Model file for the job. Use its own axes, mm. Face numbers are marked on the shaded views. A direction names the side the tool comes from. Coordinates: 2 decimals unless noted, no trailing zeros. Order: outer loops, then holes, each group sorted by start corner. A loop starts at its lowest first (then second) coordinate and runs counter-clockwise, first axis right, second up. Notation, with made-up numbers: (-25, 60) -> (-9, 60) arc R28 cw to (-9, 95) -> close; hole circle Ø3 at (24, 17). An arc over 180 degrees is marked (long way). Use CSV: the item, a comma, the result in double quotes. Start each with the question number.
(1) Tool access for the marked faces 4 and 5: list every direction of +Z, -Z, +X, -X, +Y, -Y with a clear straight run to the whole face (end or side of a thin tool).
(2) Cut at D-D on x = 1. Write the cut outline in (y, z) (3 decimals).
(3) Cut at C-C on z = 0. Write the cut outline in (x, y) (3 decimals), plus the area to 3 significant figures.
(4) Probe L1, parallel to Z at x = 0, y = 0.2; L2, parallel to X at y = 0.2, z = 0; L3, parallel to Y at x = 0.75, z = -1.1. List the from-to ranges inside material, lowest first.
(5) Pull direction Z, two halves, no side cores. Call the marked faces 1, 2 and 3: pulls with the +Z half, pulls with the -Z half, needs draft (parallel to the pull), parting line crosses it, or undercut.
(6) Cut at A-A on x = 0. Write the cut outline in (y, z) (3 decimals), plus the area to 3 significant figures.
```python
from build123d import *

# Parameters (mm, degrees)
BOSS_EXTRUDE1_DEPTH   = 2
BOSS_EXTRUDE1_2_DEPTH = 2
BOSS_EXTRUDE2_DEPTH   = 0.5
HOLE2_OUTLINE_R       = 0.5
HOLE2_DEPTH           = 0.5
FILLET2_R             = 0.125
FILLET3_R             = 0.125


# Read off the part's stored shape, not the designer's step: Hole2
with BuildPart() as part:
    # Sketch1 → Boss-Extrude1 (new body)
    with BuildSketch(Plane(origin=(0, 0, 0), x_dir=(1, 0, 0), z_dir=(0, 1, 0))):
        with BuildLine():
            Line((-1.0392304845412224, 2.6), (-1.5, 2.6))
            ThreePointArc((-1.5, 2.6), (-4.1, -1.7e-16), (-1.4999999999999993, -2.6))
            Line((-1.5, -2.6), (-1.039230484541227, -2.6))
            ThreePointArc((-1.0392304845412341, -2.6000000000000365), (-2.8, 2.83e-15), (-1.0392304845412292, 2.6000000000000387))
        make_face()
    extrude(amount=BOSS_EXTRUDE1_DEPTH)



with BuildPart() as body_2:
    # Sketch1 → Boss-Extrude1 2 (new body)
    with BuildSketch(Plane(origin=(0, 0, 0), x_dir=(1, 0, 0), z_dir=(0, 1, 0))):
        with BuildLine():
            Line((1.4999999999999991, 2.6000000000000005), (1.039230484541188, 2.6000000000000005))
            ThreePointArc((1.0392304845411973, 2.6000000000000516), (2.8000000000000003, 3.11e-15), (1.039230484541203, -2.6000000000000494))
            Line((1.0392304845411937, -2.5999999999999996), (1.5000000000000009, -2.5999999999999996))
            ThreePointArc((1.5000000000000009, -2.5999999999999996), (4.1, 1.73e-15), (1.4999999999999984, 2.6000000000000005))
        make_face()
    extrude(amount=BOSS_EXTRUDE1_2_DEPTH)


with BuildPart() as part_1:
    add(part.part)

    add(body_2.part)  # Boss-Extrude2 merges body 2
    # Sketch1<3> → Boss-Extrude2 (add)
    with BuildSketch(Plane(origin=(0, 0, 0), x_dir=(1, 0, 0), z_dir=(0, 1, 0))):
        with BuildLine():
            Line((1.0392304845411884, 2.6000000000000005), (-1.0392304845412224, 2.6))
            ThreePointArc((-1.0392304845412292, 2.6000000000000387), (-2.8, 2.83e-15), (-1.0392304845412341, -2.6000000000000365))
            Line((-1.039230484541227, -2.6), (1.0392304845411937, -2.5999999999999996))
            ThreePointArc((1.039230484541203, -2.600000000000049), (2.3183879481997147, -1.5700564708450193), (2.8, -6.9e-16))
            ThreePointArc((2.8, 0), (2.318387948199713, 1.5700564708450213), (1.0392304845411973, 2.6000000000000516))
        make_face()
    extrude(amount=BOSS_EXTRUDE2_DEPTH)

    # Hole2 outline → Hole2 (cut)
    with BuildSketch(Plane(origin=(0, 0, 0), x_dir=(1, 0, 0), z_dir=(0, 1, 0))):
        Circle(HOLE2_OUTLINE_R)
    extrude(amount=HOLE2_DEPTH, mode=Mode.SUBTRACT)

    # Fillet2
    # the kernel refuses this fillet: 0.125 mm, written as the material it takes off along each edge
    with BuildSketch(Plane(origin=(1.4999999999999987, 0, -2.6000000000000005), x_dir=(0, 1, 3.55e-15), z_dir=(-1, 0, 1.5e-16))) as fillet2_piece_1:
        with BuildLine():
            CenterArc((FILLET2_R, -FILLET2_R), FILLET2_R, 90.00000000000021, 89.99999999999979)
            Line((4.3e-16, -FILLET2_R), (0, 0))
            Line((0, 0), (FILLET2_R, 0))
        make_face()
    extrude(amount=2.9999999999999987, mode=Mode.SUBTRACT)
    with BuildSketch(Plane(origin=(1.4999999999999996, 0, -3.3e-16), x_dir=(5.1e-16, 0, 1), z_dir=(-1, 0, 5.1e-16))) as fillet2_piece_2:
        with BuildLine():
            CenterArc((2.6 - FILLET2_R, FILLET2_R), FILLET2_R, 270, 90)
            Line((2.6, FILLET2_R), (2.6, 0))
            Line((2.6, 0), (2.6 - FILLET2_R, 0))
        make_face()
    revolve(axis=Axis((1.4999999999999996, 0, -3.3e-16), (0, 1, 0)), revolution_arc=180, mode=Mode.SUBTRACT)
    with BuildSketch(Plane(origin=(1.5000000000000009, 0, 2.5999999999999996), x_dir=(-1.5e-16, 0, -1), z_dir=(-1, 0, 1.5e-16))) as fillet2_piece_3:
        with BuildLine():
            CenterArc((FILLET2_R, -FILLET2_R), FILLET2_R, 90, 90)
            Line((0, -FILLET2_R), (0, 0))
            Line((0, 0), (FILLET2_R, 0))
        make_face()
    extrude(amount=3.0000000000000004, mode=Mode.SUBTRACT)
    with BuildSketch(Plane(origin=(-1.0392304845412306, 0.5, 2.6000000000000183), x_dir=(-0.8909362232588717, 0, -0.4541284466813525), z_dir=(0, 1, 0))) as fillet2_piece_4:
        with BuildLine():
            CenterArc((0.5210688048998693, 0.1244811743822189), FILLET2_R, 115.6197462863135, 149.1581720450634)
            Line((0.4670192388207316, 0.23719161935808136), (0.46161428221281786, 0.24846266385566762))
            ThreePointArc((0.46161428221281786, 0.24846266385566762), (0.404839646312147, 0.2203852471241299), (-0.00567660558351699, 0.01113670279073605))
            Line((-0.00567660558351699, 0.01113670279073605), (0.00113770481419139, -0.01244811743822212))
            ThreePointArc((0.00113770481419139, -0.01244811743822212), (0.254845878378973, -0.00087830616170155), (0.5085540519437544, -0.0124481174382219))
            Line((0.5085540519437544, -0.0124481174382219), (0.5096917567579465, -1e-17))
        make_face()
    extrude(amount=2.809500939581575, mode=Mode.SUBTRACT)
    with BuildSketch(Plane(origin=(1.0392304845411986, 0.5, 2.600000000000024), x_dir=(0.8909362232588801, 0, -0.45412844668133606), z_dir=(0, 1, 0))) as fillet2_piece_5:
        with BuildLine():
            CenterArc((0.5210688048999061, -0.12448117438221841), FILLET2_R, 95.22208166862436, 149.158172045063)
            Line((0.4670192388207701, -0.23719161935808164), (0.46161428221285655, -0.248462663855668))
            ThreePointArc((0.46161428221285655, -0.248462663855668), (0.4048396463121838, -0.22038524712413216), (-0.00567660558351678, -0.01113670279073616))
            Line((-0.00567660558351678, -0.01113670279073616), (0.00113770481419136, 0.01244811743822204))
            ThreePointArc((0.00113770481419136, 0.01244811743822204), (0.2548458783789898, 0.00087830616169669), (0.5085540519437883, 0.0124481174382219))
            Line((0.5085540519437883, 0.0124481174382219), (0.5096917567579807, 2e-17))
        make_face()
    extrude(amount=2.8095009395816612, mode=Mode.SUBTRACT)
    with BuildSketch(Plane(origin=(1.0392304845411924, 0.5, -2.600000000000026), x_dir=(0.9999989359619427, 0, 0.001458792302720678), z_dir=(0, 1, 0))) as fillet2_piece_6:
        with BuildLine():
            CenterArc((0.5209523714738641, -0.12496755127300935), FILLET2_R, 88.69445799122111, 149.1581720450468)
            Line((0.45444002573679215, -0.23080283775418345), (0.447788791163085, -0.24138636640230085))
            ThreePointArc((0.447788791163085, -0.24138636640230085), (0.22682229100640774, -0.11618451467849848), (-0.00462248445880959, -0.01161389845952106))
            Line((-0.00462248445880959, -0.01161389845952106), (-1.823490378401e-05, 0.01249998669952446))
            ThreePointArc((-1.823490378401e-05, 0.01249998669952446), (0.46075079027872196, 0.01317215372197879), (0.5240851762685466, 0.01249675512730089))
            Line((0.5240851762685466, 0.01249675512730089), (0.5238003758326663, 0))
        make_face()
    extrude(amount=2.8095009395816657, mode=Mode.SUBTRACT)
    with BuildSketch(Plane(origin=(-1.4999999999999996, 0, 0), x_dir=(-1.7e-16, 0, -1), z_dir=(1, 0, -1.7e-16))) as fillet2_piece_7:
        with BuildLine():
            CenterArc((2.6 - FILLET2_R, FILLET2_R), FILLET2_R, 270, 90)
            Line((2.6 - FILLET2_R, -1e-17), (2.6, 0))
            Line((2.6, 0), (2.6, FILLET2_R))
        make_face()
    revolve(axis=Axis((-1.4999999999999996, 0, 0), (0, 1, 0)), revolution_arc=180, mode=Mode.SUBTRACT)
    with BuildSketch(Plane(origin=(-1.0392304845412257, 0.5, -2.600000000000019), x_dir=(-0.9999989359619427, 0, 0.0014587923027088937), z_dir=(0, 1, 0))) as fillet2_piece_8:
        with BuildLine():
            CenterArc((0.5209523714738317, 0.1249675512730093), FILLET2_R, 122.14736996373313, 149.15817204504657)
            Line((0.4544400257367579, 0.23080283775418217), (0.44778879116305065, 0.24138636640229952))
            ThreePointArc((0.44778879116305065, 0.24138636640229952), (0.2268222910063884, 0.11618451467850208), (-0.00462248445880995, 0.01161389845952101))
            Line((-0.00462248445880995, 0.01161389845952101), (-1.823490378386e-05, -0.01249998669952446))
            ThreePointArc((-1.823490378386e-05, -0.01249998669952446), (0.46075079027869037, -0.01317215372197953), (0.524085176268516, -0.01249675512730089))
            Line((0.524085176268516, -0.01249675512730089), (0.5238003758326356, 0))
        make_face()
    extrude(amount=2.809500939581589, mode=Mode.SUBTRACT)

    # Fillet3
    fillet3_edges = [part_1.edges().sort_by_distance(p)[0] for p in [
        (4.1, 2, 5.853e-14),
        (-2.799999999999999, 2, -1.78e-15),
        (-4.1, 2, 6.033e-14),
        (-1.440341394717322, 2, -2.510422560661599),
        (-1.4403413947172043, 2, 2.5104225606616026),
        (2.8, 2, -2.2e-16),
        (1.4403413947173214, 2, -2.5104225606615973),
        (1.4403413947172052, 2, 2.510422560661605),
    ]]
    fillet(fillet3_edges, radius=FILLET3_R)


solid = part_1.part
```
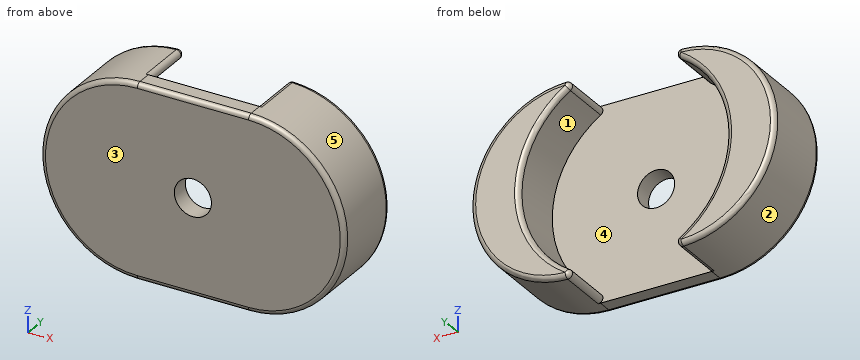
Outcome:
1,face 4,"+Y"
1,face 5,"+X, +Y, -Y"
2,outline,"(0, -2.475) arc R0.125 ccw to (0.125, -2.6) -> (0.5, -2.6) -> (0.5, 2.6) -> (0.125, 2.6) arc R0.125 ccw to (0, 2.475) -> close"
3,outline,"(-4.1, 0.125) arc R0.125 ccw to (-3.975, 0) -> (-0.5, 0) -> (-0.5, 0.5) -> (-2.8, 0.5) -> (-2.8, 1.875) arc R0.125 ccw to (-2.925, 2) -> (-3.975, 2) arc R0.125 ccw to (-4.1, 1.875) -> close; (0.5, 0) -> (3.975, 0) arc R0.125 ccw to (4.1, 0.125) -> (4.1, 1.875) arc R0.125 ccw to (3.975, 2) -> (2.925, 2) arc R0.125 ccw to (2.8, 1.875) -> (2.8, 0.5) -> (0.5, 0.5) -> close"
3,area,"7.48 mm2"
4,L1,"-2.6 to -0.5, 0.5 to 2.6"
4,L2,"-4.1 to -0.5, 0.5 to 4.1"
4,L3,"0 to 0.5"
5,face 1,"undercut"
5,face 2,"parting line crosses it"
5,face 3,"needs draft"
6,outline,"(0, -2.475) arc R0.125 ccw to (0.125, -2.6) -> (0.5, -2.6) -> (0.5, -0.5) -> (0, -0.5) -> close; (0, 0.5) -> (0.5, 0.5) -> (0.5, 2.6) -> (0.125, 2.6) arc R0.125 ccw to (0, 2.475) -> close"
6,area,"2.09 mm2"
